Design review of the part built by this model. Coordinates are the model's own, in mm. A direction names the side the tool comes from. Round coordinates to 2 decimals unless told otherwise and drop trailing zeros. Order: outer loops, then holes, each group sorted by start corner. A loop starts at its lowest first (then second) coordinate and runs counter-clockwise, first axis right, second up.
Autodesk Inventor part; units mm, degrees
ref_plane "YZ Plane" through (0, 0, 0) normal (1, 0, 0) x (0, 1, 0)
ref_plane "XZ Plane" through (0, 0, 0) normal (0, 1, 0) x (-1, 0, 0)
ref_plane "XY Plane" through (0, 0, 0) normal (0, 0, 1) x (1, 0, 0)
sketch "Sketch1" plane through (0, 0, 0) normal (0, 0, 1) x (1, 0, 0)
  line L0 (-30.479, 15.7185) -> (11.521, 15.7185)
  line L1 (11.521, 15.7185) -> (11.521, 11.2185)
  line L2 (11.521, 11.2185) -> (-30.479, 11.2185)
  line L3 (-30.479, 11.2185) -> (-30.479, 15.7185)
  line L4 (-30.479, 11.2185) -> (-1.479, 11.2185)
  line L5 (-1.479, 11.2185) -> (-1.479, 3.2185)
  line L6 (-1.479, 3.2185) -> (-30.479, 3.2185)
  line L7 (-30.479, 3.2185) -> (-30.479, 11.2185)
  point P0 (0, 0)
  point P1 (-1.479, 11.2185)
  dimension "d0" = 42
  dimension "d1" = 4.5
  dimension "d2" = 29
  dimension "d3" = 8
extrude "Extrusion1" add sketch "Sketch1" along normal blind 8.5
sketch "Sketch2" plane through (0, 0, 8.5) normal (0, 0, 1) x (1, 0, 0)
  line L0 (-30.479, 15.7185) -> (-30.479, 3.2185)
  line L1 (-30.479, 15.7185) -> (16.521, 15.7185)
  line L2 (16.521, 15.7185) -> (16.521, -16.2815)
  line L3 (16.521, -16.2815) -> (-30.479, -16.2815)
  line L4 (-30.479, -16.2815) -> (-30.479, 15.7185)
  point P0 (0, 0)
  dimension "d6" = 47
  dimension "d7" = 32
extrude "Extrusion2" add sketch "Sketch2" along normal blind 1.2
sketch "Sketch3" plane through (0, 0, 8.5) normal (0, 0, -1) x (-1, 0, 0)
  line L0 (30.479, 3.2185) -> (30.479, -16.2815)
  line L1 (30.479, -6.2815) -> (15.479, -6.2815)
  line L2 (15.479, -6.2815) -> (15.479, -13.2815)
  line L3 (15.479, -13.2815) -> (30.479, -13.2815)
  line L4 (30.479, -13.2815) -> (30.479, -6.2815)
  line L5 (30.479, -16.2815) -> (-16.521, -16.2815)
  point P0 (0, 0)
  dimension "d10" = 3
  dimension "d11" = 7
  dimension "d12" = 15
extrude "Extrusion3" add sketch "Sketch3" along normal blind 8.5
sketch "Sketch4" plane through (0, 0, 8.5) normal (0, 0, -1) x (-1, 0, 0)
  line L0 (-16.521, -16.2815) -> (-16.521, 15.7185)
  line L1 (-16.521, -1.2815) -> (-9.521, -1.2815)
  line L2 (-9.521, -1.2815) -> (-9.521, -11.2815)
  line L3 (-9.521, -11.2815) -> (-16.521, -11.2815)
  line L4 (-16.521, -11.2815) -> (-16.521, -1.2815)
  line L5 (30.479, -16.2815) -> (-16.521, -16.2815)
  point P0 (0, 0)
  dimension "d15" = 7
  dimension "d16" = 10
  dimension "d17" = 5
extrude "Extrusion4" add sketch "Sketch4" along normal blind 8.5
sketch "Sketch5" plane through (0, 0, 0) normal (0, 0, -1) x (-1, 0, 0)
  line L0 (-16.521, 15.7185) -> (30.479, 15.7185)
  line L1 (30.479, 3.2185) -> (1.479, 3.2185)
  line L2 (30.479, 15.7185) -> (20.479, 15.7185)
  line L3 (20.479, 15.7185) -> (20.479, 3.2185)
  line L4 (20.479, 3.2185) -> (30.479, 3.2185)
  line L5 (30.479, 3.2185) -> (30.479, 15.7185)
  point P0 (0, 0)
  dimension "d20" = 10
extrude "Extrusion5" cut sketch "Sketch5" against normal blind 8.5
sketch "Sketch6" plane through (0, 0, 0) normal (0, 0, -1) x (-1, 0, 0)
  line L0 (15.479, -6.2815) -> (30.479, -6.2815)
  line L1 (15.479, -6.2815) -> (30.479, -6.2815)
  line L2 (30.479, -6.2815) -> (30.479, -9.2815)
  line L3 (30.479, -9.2815) -> (15.479, -9.2815)
  line L4 (15.479, -9.2815) -> (15.479, -6.2815)
  line L5 (30.479, -13.2815) -> (30.479, -6.2815)
  point P0 (0, 0)
  dimension "d23" = 3
extrude "Extrusion6" cut sketch "Sketch6" against normal blind 8.5
sketch "Sketch7" plane through (0, 0, 8.5) normal (0, 0, -1) x (-1, 0, 0)
  line L0 (-16.521, 15.7185) -> (30.479, 15.7185)
  line L1 (20.479, 15.7185) -> (30.479, 15.7185)
  line L2 (30.479, 15.7185) -> (30.479, 3.2185)
  line L3 (30.479, 3.2185) -> (20.479, 3.2185)
  line L4 (20.479, 3.2185) -> (20.479, 15.7185)
  line L5 (20.479, 3.2185) -> (1.479, 3.2185)
  line L6 (30.479, 15.7185) -> (30.479, -9.2815)
  line L7 (20.479, 3.2185) -> (20.479, 15.7185)
  point P0 (0, 0)
extrude "Extrusion7" cut sketch "Sketch7" against normal blind 8.5
chamfer "Chamfer1" distance 5 angle 45 1 edges at (-20.479, 3.2185, 9.1)
properties part number "PD board supporter"
1) Clearance check with flat-ended pins moving along their axes: P1, Ø1.5, axis at x = 1, z = 4, coming from the -Y side; P2, Ø1, axis at x = -28, z = 9, coming from the +Y side; P3, Ø2.5, axis at y = -7, z = 3, coming from the -X side. State where each tip first meets the part, or that it passes through.
Results:
P1: stops at y = 11.22
P2: stops at y = 3.22
P3: stops at x = 9.52
2) To check wall thickness, follow line 1 along Y through (x, z) = (-4.5, 2); line 2 along Z through (x, y) = (-2.5, -2.5); line 3 along X through (y, z) = (-3, 2). State the ranges of each line that lie inside material, in increasing order.
Results:
line 1: y = 3.22 to 15.72
line 2: z = 8.5 to 9.7
line 3: x = 9.52 to 16.52
3) The part is to be moulded in two halves that separate along Y. For faces 1 (the face through (13, -1.282, 4)), 2 (the face through (-23, -13.282, 4)), 3 (the face through (-1.479, 7, 4)), say which applies: released by +Y, released by -Y, zero draft, split by the parting line, or undercut.
Results:
face 1: undercut
face 2: released by -Y
face 3: zero draft
4) For faces 4 (the face through (-20.479, 10, 5)), 5 (the face through (9.521, -6, 4)), 6 (the face through (-11, 3.218, 4)), list the 3-axis set-ups (+Z, -Z, +X, -X, +Y, -Y) from which the entire face can be reached by the end or side of a thin tool; tool diameter is ignored.
Results:
face 4: -Z, -X, +Y
face 5: -Z, -Y
face 6: -Z, +X, -X
5) Take a section at D-D on x = 1. Give the boundary of the cut face in (y, z), plus the area to 4 significant figures.
Results:
outline: (-16.28, 8.5) - (11.22, 8.5) - (11.22, 0) - (15.72, 0) - (15.72, 9.7) - (-16.28, 9.7) - close
area: 76.65 mm2
6) Take a section at A-A on z = 7. Give the boundary of the cut face in (x, y), plus the area to 3 significant figures.
Results:
outline: (-30.48, -13.28) - (-15.48, -13.28) - (-15.48, -9.28) - (-30.48, -9.28) - close; (-20.48, 3.22) - (-1.48, 3.22) - (-1.48, 11.22) - (11.52, 11.22) - (11.52, 15.72) - (-20.48, 15.72) - close; (9.52, -11.28) - (16.52, -11.28) - (16.52, -1.28) - (9.52, -1.28) - close
area: 426 mm2
7) Take a section at B-B on x = -27. Give the boundary of the cut face in (y, z), plus the area to 3 significant figures.
Results:
outline: (-16.28, 8.5) - (-13.28, 8.5) - (-13.28, 0) - (-9.28, 0) - (-9.28, 8.5) - (3.22, 8.5) - (3.22, 9.7) - (-16.28, 9.7) - close
area: 57.4 mm2
8) Take a section at C-C on y = -7. Give the boundary of the cut face in (x, z), plus the area to 3 significant figures.
Results:
outline: (-30.48, 8.5) - (9.52, 8.5) - (9.52, 0) - (16.52, 0) - (16.52, 9.7) - (-30.48, 9.7) - close
area: 116 mm2
